Here's how the part is built. I have some questions about the finished solid (model axes, mm). A direction names the side the tool comes from. Round coordinates to 2 decimals unless told otherwise and drop trailing zeros. Order: outer loops, then holes, each group sorted by start corner. A loop starts at its lowest first (then second) coordinate and runs counter-clockwise, first axis right, second up. Notation, with made-up numbers: (88, 24.5) - (105, 24.5) arc R18 ccw to (105, 30.5) - close; hole circle Ø3 at (-19, 44). An arc over 180 degrees is marked (long way). One line per item, written item: value.
from build123d import *

# Parameters (mm, degrees)
SKETCH1_R           = 2.5
BOSS_EXTRUDE1_DEPTH = 8
FILLET1_R           = 1
FILLET2_R           = 2


with BuildPart() as part:
    # Sketch1 → Boss-Extrude1 (new body)
    with BuildSketch(Plane.XY):
        with BuildLine():
            Line((-0.448423134, -12.085069991), (2.54016096, -11.823602763))
            Line((2.54016096, -11.823602763), (2.365849475, -9.831213367))
            Line((2.365849475, -9.831213367), (15, -1.5))
            Line((15, -1.5), (18, -1.5))
            Line((18, -1.5), (18, 1.5))
            Line((18, 1.5), (3.708099244, 1.5))
            ThreePointArc((3.708099244, 1.5), (-2.949109347, 2.70236083), (-1.171109903, -3.824722421))
            Line((-1.171109903, -3.824722421), (-0.448423134, -12.085069991))
        make_face()
        Circle(SKETCH1_R, mode=Mode.SUBTRACT)
    extrude(amount=BOSS_EXTRUDE1_DEPTH)

    # Fillet1
    fillet1_edges = [part.edges().sort_by_distance(p)[0] for p in [
        (2.54016096, -11.823602763, 4),
        (18, -1.5, 4),
        (-0.448423134, -12.085069991, 4),
    ]]
    fillet(fillet1_edges, radius=FILLET1_R)

    # Fillet2
    fillet2_edges = [part.edges().sort_by_distance(p)[0] for p in [
        (18, 1.5, 4),
    ]]
    fillet(fillet2_edges, radius=FILLET2_R - 0.0001)  # a hair under: the kernel refuses the full size


solid = part.part
Q1. If we section it at B-B, the plane x = 0.25: Please give me the cut outline in (y, z).
Results list:
outline: (-11.98, 0) - (-2.49, 0) - (-2.49, 8) - (-11.98, 8) - close; (2.49, 0) - (3.99, 0) - (3.99, 8) - (2.49, 8) - close
Q2. If we section it at A-A, the plane y = 0: Please give me the cut outline in (x, z), then the cut area to 3 significant figures.
Results list:
outline: (-4, 0) - (-2.5, 0) - (-2.5, 8) - (-4, 8) - close; (2.5, 0) - (17.94, 0) - (17.94, 8) - (2.5, 8) - close
area: 135 mm²
Q3. We'd pull the mould along X, two halves only. Please class faces 1 (the flat face through (8.594, -5.724, 3.944)), 2 (the flat face through (10, 1.5, 4)), 3 (the cylindrical face through (-0.54, -2.44, 3.94)): released by +X, released by -X, zero draft, split by the parting line, or undercut.
Results list:
face 1: released by +X
face 2: zero draft
face 3: undercut
Q4. Which directions (+Z, -Z, +X, -X, +Y, -Y) give clear straight access to the entire face, cutting with the end or side of a thin tool? Please do faces 4 (the flat face through (2.41, -10.34, 3.94)), 5 (the flat face through (-0.858, -7.406, 3.944)), 6 (the flat face through (16, -1.5, 4)).
Results list:
face 4: +Z, -Z, +X
face 5: +Z, -Z, -X, -Y
face 6: +Z, -Z, +X, -Y
Q5. Will these pins go through, and if not, where does the flat tip stop? pin 1 (1.6 mm diameter, centred on x = 16, z = 5, fed in from -Y); pin 2 (3 mm diameter, centred on x = 13.5, z = 3.5, fed in from -Y); pin 3 (1.5 mm diameter, centred on y = -7, z = 2.5, fed in from -X); pin 4 (3 mm diameter, centred on x = 0, y = 0, fed in from -Z).
Results list:
pin 1: y = -1.5
pin 2: y = -3.48
pin 3: x = -0.96
pin 4: through
Q6. If we section it at D-D, the plane x = 7.5: Please give me the cut outline in (y, z).
Results list:
outline: (-6.45, 0) - (1.5, 0) - (1.5, 8) - (-6.45, 8) - close
Q7. If I drill on line 1 along X through (y, z) = (-2.25, 0.5); line 2 along Y through (x, z) = (2.25, 7); line 3 along Y through (x, z) = (15, 6.5), over which ranges is the centre line in solid material (lowest first)?
Results list:
line 1: -3.31 to -1.09, 1.09 to 13.86
line 2: -11.52 to -1.09, 1.09 to 3.31
line 3: -1.5 to 1.5
